Build history of the part. All positions in model axes, mm. Face numbers are marked on the shaded views. Round coordinates to 2 decimals unless told otherwise and drop trailing zeros. Write each loop counter-clockwise with the first axis right and the second up, starting at its lowest first coordinate (ties: lowest second). Pieces come first, ordered by that corner, then holes. Notation, with made-up numbers: (26, -30.75) -> (57, -30.75) arc R20 cw to (57, 7.25) -> close; hole circle Ø1 at (57, 72). An arc over 180 degrees is marked (long way). Return JSON: item names as keys, results as strings.
from build123d import *

# Parameters (mm, degrees)
BOSS_EXTRUDE1_DEPTH     = 508.5
CUT_EXTRUDE4_REACH      = 518.756
CUT_EXTRUDE4_END_RADIUS = 90
SKETCH6_R               = 5.565
CUT_EXTRUDE2_REACH      = 520.673
CUT_EXTRUDE2_END_RADIUS = 90
SKETCH3_R               = 5.565
CUT_EXTRUDE3_REACH      = 520.673
CUT_EXTRUDE3_END_RADIUS = 90
SKETCH5_R               = 5.565
LPATTERN2_COUNT         = 2
LPATTERN2_PITCH         = 485.5
CUT_EXTRUDE5_DEPTH      = 20


with BuildPart() as part:
    # Sketch1 → Boss-Extrude1 (new body)
    with BuildSketch(Plane(origin=(0, 0, 0), x_dir=(1, 0, 0), z_dir=(0, 1, 0))):
        with BuildLine():
            Line((0, 92), (0, 90))
            ThreePointArc((0, 90), (63.639610307, 63.639610307), (90, 0))
            Line((90, 0), (92, 0))
            ThreePointArc((92, 0), (65.053823869, 65.053823869), (0, 92))
        make_face()
    extrude(amount=BOSS_EXTRUDE1_DEPTH)

    # Cut-Extrude4: up to this cylinder (the profile starts outside it)
    cut_extrude4_end = Plane(origin=(0, 10, 0), z_dir=(0, -1, 0)) * Cylinder(CUT_EXTRUDE4_END_RADIUS, 1218.512, mode=Mode.PRIVATE)
    # Sketch6 → Cut-Extrude4 (cut, up to the surface)
    with BuildSketch(Plane(origin=(65.053823869, 0, -65.053823869), x_dir=(-0.7071067811865486, 0, -0.7071067811865465), z_dir=(0.7071067811865465, 0, -0.7071067811865486)), mode=Mode.PRIVATE) as cut_extrude4_sk1:
        with Locations((0, 10)):
            Circle(SKETCH6_R)
    cut_extrude4_tool1 = extrude(cut_extrude4_sk1.sketch, amount=-CUT_EXTRUDE4_REACH, mode=Mode.PRIVATE) - cut_extrude4_end
    add(cut_extrude4_tool1.solids().sort_by_distance((65.053824, 10, -65.053824))[0], mode=Mode.SUBTRACT)

    # Cut-Extrude2: up to this cylinder (the profile starts outside it)
    cut_extrude2_end = Plane(origin=(0, 10, 0), z_dir=(0, -1, 0)) * Cylinder(CUT_EXTRUDE2_END_RADIUS, 1222.346, mode=Mode.PRIVATE)
    # Sketch3 → Cut-Extrude2 (cut, up to the surface)
    with BuildSketch(Plane(origin=(84.996916991, 0, -35.206875778), x_dir=(-0.38268343236509045, 0, -0.9238795325112865), z_dir=(0.9238795325112865, 0, -0.38268343236509045)), mode=Mode.PRIVATE) as cut_extrude2_sk1:
        with Locations((0, 10)):
            Circle(SKETCH3_R)
    cut_extrude2_tool1 = extrude(cut_extrude2_sk1.sketch, amount=-CUT_EXTRUDE2_REACH, mode=Mode.PRIVATE) - cut_extrude2_end
    cut_extrude2 = cut_extrude2_tool1.solids().sort_by_distance((84.996917, 10, -35.206876))[0]
    add(cut_extrude2, mode=Mode.SUBTRACT)

    # Cut-Extrude3: up to this cylinder (the profile starts outside it)
    cut_extrude3_end = Plane(origin=(0, 10, 0), z_dir=(0, -1, 0)) * Cylinder(CUT_EXTRUDE3_END_RADIUS, 1222.346, mode=Mode.PRIVATE)
    # Sketch5 → Cut-Extrude3 (cut, up to the surface)
    with BuildSketch(Plane(origin=(35.206875778, 0, -84.996916991), x_dir=(-0.9238795325112878, 0, -0.3826834323650876), z_dir=(0.3826834323650876, 0, -0.9238795325112878)), mode=Mode.PRIVATE) as cut_extrude3_sk1:
        with Locations((0, 10)):
            Circle(SKETCH5_R)
    cut_extrude3_tool1 = extrude(cut_extrude3_sk1.sketch, amount=-CUT_EXTRUDE3_REACH, mode=Mode.PRIVATE) - cut_extrude3_end
    cut_extrude3 = cut_extrude3_tool1.solids().sort_by_distance((35.206876, 10, -84.996917))[0]
    add(cut_extrude3, mode=Mode.SUBTRACT)

    # LPattern2: Cut-Extrude2, Cut-Extrude3 ×2
    with Locations(*[(0, i * LPATTERN2_PITCH, 0) for i in range(1, LPATTERN2_COUNT)]):
        add(cut_extrude2, mode=Mode.SUBTRACT)
        add(cut_extrude3, mode=Mode.SUBTRACT)

    # Sketch7 → Cut-Extrude5 (cut)
    with BuildSketch(Plane.XZ):
        with BuildLine():
            ThreePointArc((90, 0), (86.112133982, -26.166780106), (74.784435976, -50.072828318))
            Line((74.784435976, -50.072828318), (76.447375943, -51.183969281))
            ThreePointArc((76.447375943, -51.183969281), (88.026014867, -26.747349525), (92, 0))
            Line((92, 0), (90, 0))
        make_face()
        with BuildLine():
            Line((51.183969281, -76.447375943), (50.072828318, -74.784435976))
            ThreePointArc((50.072828318, -74.784435976), (26.166780106, -86.112133982), (0, -90))
            Line((0, -90), (0, -92))
            ThreePointArc((0, -92), (26.747349525, -88.026014867), (51.183969281, -76.447375943))
        make_face()
    extrude(amount=-CUT_EXTRUDE5_DEPTH, mode=Mode.SUBTRACT)


solid = part.part
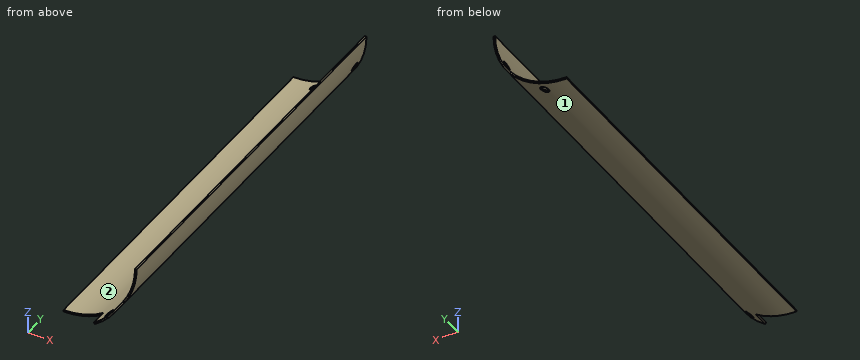
Q1. Pin check, flat tips, straight feed: pin 1 Ø5 at (y, z) = (238, -74) entering from -X; pin 2 Ø8.5 at (x, z) = (31.5, -84) entering from -Y; pin 3 Ø6 at (x, y) = (23, 240) entering from +Z. Stop position of each tip, or through.
Verdict:
{"pin 1": "stops at x = 47.41", "pin 2": "stops at y = 20", "pin 3": "stops at z = -86.16"}
Q2. Saw through at A-A on y = 226. List the corners of the cut face in (x, z).
Verdict:
{"outline": "(0, -92) arc R92 ccw to (92, 0) -> (90, 0) arc R90 cw to (0, -90) -> close"}
Q3. Saw through at B-B on x = 7.5. List the corners of the cut face in (y, z).
Verdict:
{"outline": "(20, -91.69) -> (508.5, -91.69) -> (508.5, -89.69) -> (20, -89.69) -> close"}
Q4. Two-plate mould, pull along X, no slides. Class the marked faces 1 and 2: +X half, -X half, draft (parallel to the pull), parting line (faces both ways), or undercut.
Verdict:
{"face 1": "+X half", "face 2": "-X half"}
Q5. Wall check: L1, parallel to Z at x = 45, y = 193; L2, parallel to X at y = 79, z = -63; L3, parallel to X at y = 404, z = -83.5. Give the ranges that are in metal, low to high.
Verdict:
{"L1": "z = -80.24 to -77.94", "L2": "x = 64.27 to 67.04", "L3": "x = 33.58 to 38.62"}
